Autodesk Inventor part; units mm, degrees
ref_plane "YZ Plane" through (0, 0, 0) normal (1, 0, 0) x (0, 1, 0)
ref_plane "XZ Plane" through (0, 0, 0) normal (0, 1, 0) x (-1, 0, 0)
ref_plane "XY Plane" through (0, 0, 0) normal (0, 0, 1) x (1, 0, 0)
sketch "Sketch1" plane through (0, 0, 0) normal (0, 1, 0) x (-1, 0, 0)
  line L0 (7.5, 50) -> (-7.5, 50)
  line L1 (-7.5, 50) -> (-7.5, -50)
  line L2 (-7.5, -50) -> (7.5, -50)
  line L3 (7.5, -50) -> (7.5, 50) construction
  line L4 (7.5, 50) -> (-7.5, -50) construction
  line L5 (-7.5, 50) -> (7.5, -50) construction
  line L6 (7.5, 50) -> (7.5, 45)
  line L7 (7.5, 35) -> (-4.5, 35)
  line L8 (-4.5, 35) -> (-4.5, 45)
  line L9 (-4.5, 45) -> (7.5, 45)
  line L10 (7.5, 19) -> (-4.5, 19)
  line L11 (-4.5, 19) -> (-4.5, 29)
  line L12 (-4.5, 29) -> (7.5, 29)
  line L13 (7.5, 3) -> (-4.5, 3)
  line L14 (-4.5, 3) -> (-4.5, 13)
  line L15 (-4.5, 13) -> (7.5, 13)
  line L16 (7.5, -13) -> (-4.5, -13)
  line L17 (-4.5, -13) -> (-4.5, -3)
  line L18 (-4.5, -3) -> (7.5, -3)
  line L19 (7.5, -29) -> (-4.5, -29)
  line L20 (-4.5, -29) -> (-4.5, -19)
  line L21 (-4.5, -19) -> (7.5, -19)
  line L22 (7.5, -45) -> (-4.5, -45)
  line L23 (-4.5, -45) -> (-4.5, -35)
  line L24 (-4.5, -35) -> (7.5, -35)
  line L25 (7.5, 35) -> (7.5, 29)
  line L26 (7.5, 19) -> (7.5, 13)
  line L27 (7.5, 3) -> (7.5, -3)
  line L28 (7.5, -13) -> (7.5, -19)
  line L29 (7.5, -29) -> (7.5, -35)
  line L30 (7.5, -45) -> (7.5, -50)
  point P0 (0, 0)
  point P1 (7.5, 0)
  dimension "d0" = 15
  dimension "d1" = 100
  dimension "d4" = 5
  dimension "d5" = 10
  dimension "d6" = 12
  dimension "d9" = 16
  dimension "d14" = 10
extrude "Extrusion1" add sketch "Sketch1" along normal blind 20
properties part number "pneunet_approximate_test"
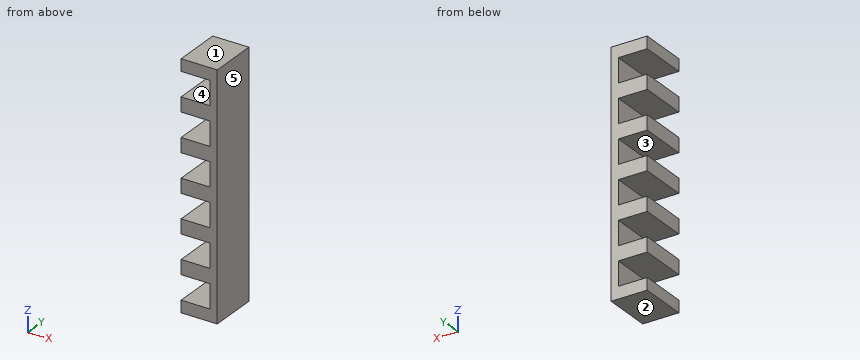
The listing builds one solid part. Answer for the finished solid, in the listing's coordinates (mm). Face numbers are marked on the shaded views. A direction names the side the tool comes from. Coordinates: 2 decimals unless noted, no trailing zeros. Loops run counter-clockwise (first coordinate to the right, second up) from the corner with the lowest first, then second, coordinate; pieces in that order, holes last. Notation, with made-up numbers: (-11.5, 54) - (7.5, 54) arc R9 cw to (7.5, 65) - close; hole circle Ø4 at (-28.75, -26). An arc over 180 degrees is marked (long way). Use a Markdown table: item, result. Add a question column.
1) The mould has two halves that part along Z. Classify the marked faces 1, 2 and 3: released by +Z, released by -Z, zero draft, split by the parting line, or undercut.
2) For the marked faces 4 and 5, determine the directions among +Z, -Z, +X, -X, +Y, -Y from which every point of the face is accessible in a straight line to the end or side of a thin tool.
3) The part is cut by section C-C, the plane z = -40.5. Give the vertices of the cut face in (x, y), and give its area (3 significant figures).
4) Find the intervals of material crossed by line 1 (X direction, y = 12.5, z = 3.5), in increasing order.
5) The part is cut by section B-B, the plane y = 11.75. Give the vertices of the cut face in (x, z).
6) Given pin 1 (1.5 mm diameter, centred on y = 6, z = 4.5, fed in from -X), flat-ended and moving along its own axis, determine where the tip first touches the part or whether it passes through.
7) The part is cut by section A-A, the plane x = -3.25. Give the vertices of the cut face in (y, z).
Here are the results:
| question | item | result |
|---|---|---|
| 1 | face 1 | released by +Z |
| 1 | face 2 | released by -Z |
| 1 | face 3 | undercut |
| 2 | face 4 | -X, +Y, -Y |
| 2 | face 5 | +Z, -Z, +X, +Y, -Y |
| 3 | outline | (4.5, 0) - (7.5, 0) - (7.5, 20) - (4.5, 20) - close |
| 3 | area | 60.0 mm^2 |
| 4 | line 1 | x = 4.5 to 7.5 |
| 5 | outline | (-7.5, -50) - (7.5, -50) - (7.5, 50) - (-7.5, 50) - (-7.5, 45) - (4.5, 45) - (4.5, 35) - (-7.5, 35) - (-7.5, 29) - (4.5, 29) - (4.5, 19) - (-7.5, 19) - (-7.5, 13) - (4.5, 13) - (4.5, 3) - (-7.5, 3) - (-7.5, -3) - (4.5, -3) - (4.5, -13) - (-7.5, -13) - (-7.5, -19) - (4.5, -19) - (4.5, -29) - (-7.5, -29) - (-7.5, -35) - (4.5, -35) - (4.5, -45) - (-7.5, -45) - close |
| 6 | pin 1 | stops at x = 4.5 |
| 7 | outline | (0, -50) - (20, -50) - (20, -45) - (0, -45) - close; (0, -35) - (20, -35) - (20, -29) - (0, -29) - close; (0, -19) - (20, -19) - (20, -13) - (0, -13) - close; (0, -3) - (20, -3) - (20, 3) - (0, 3) - close; (0, 13) - (20, 13) - (20, 19) - (0, 19) - close; (0, 29) - (20, 29) - (20, 35) - (0, 35) - close; (0, 45) - (20, 45) - (20, 50) - (0, 50) - close |
